Check sheet for the modelled part. Datum: model origin and axes. Units: mm. A direction names the side the tool comes from. Coordinates: 2 decimals unless noted, no trailing zeros. Order: outer loops, then holes, each group sorted by start corner. A loop starts at its lowest first (then second) coordinate and runs counter-clockwise, first axis right, second up. Notation, with made-up numbers: (-23.75, -27) -> (8.25, -27) arc R11 cw to (8.25, -8) -> close; hole circle Ø5 at (-25, 58). An arc over 180 degrees is marked (long way). Put each result on its own line as item: value. Start each with the question number.
```python
from build123d import *

# Parameters (mm, degrees)
SKETCH1_W           = 2.8
SKETCH1_H           = 2.8
SKETCH1_W_2         = 2.7
SKETCH1_H_2         = 2.7
BOSS_EXTRUDE1_DEPTH = 3


with BuildPart() as part:
    # Sketch1 → Boss-Extrude1 (new body)
    with BuildSketch(Plane(origin=(0, 0, 0), x_dir=(1, 0, 0), z_dir=(0, 1, 0))):
        with BuildLine():
            Line((-37.844649751, 18.090932989), (-37.844649751, 15.090932989))
            Line((-37.844649751, 15.090932989), (-35.044649751, 15.090932989))
            Line((-35.044649751, 15.090932989), (-35.044649751, 12.290932989))
            Line((-35.044649751, 12.290932989), (-37.844649751, 12.290932989))
            Line((-37.844649751, 12.290932989), (-37.844649751, 6.290932989))
            Line((-37.844649751, 6.290932989), (-35.344649751, 6.290932989))
            Line((-35.344649751, 6.290932989), (-35.344649751, -53.709067011))
            Line((-35.344649751, -53.709067011), (-37.844649751, -53.709067011))
            Line((-37.844649751, -53.709067011), (-37.844649751, -71.409067011))
            ThreePointArc((-37.844649751, -71.409067011), (-25.332467624, -76.857542339), (-11.813147026, -78.719948188))
            Line((-11.813147026, -78.719948188), (-8.844649751, -78.719948188))
            Line((-8.844649751, -78.719948188), (1.155350249, -78.719948188))
            Line((1.155350249, -78.719948188), (11.155350249, -78.719948188))
            Line((11.155350249, -78.719948188), (14.123847524, -78.719948188))
            ThreePointArc((14.123847524, -78.719948188), (27.643168122, -76.857542339), (40.155350249, -71.409067011))
            Line((40.155350249, -71.409067011), (40.155350249, -53.709067011))
            Line((40.155350249, -53.709067011), (37.655350249, -53.709067011))
            Line((37.655350249, -53.709067011), (37.655350249, 6.290932989))
            Line((37.655350249, 6.290932989), (40.155350249, 6.290932989))
            Line((40.155350249, 6.290932989), (40.155350249, 12.290932989))
            Line((40.155350249, 12.290932989), (37.355350249, 12.290932989))
            Line((37.355350249, 12.290932989), (37.355350249, 15.090932989))
            Line((37.355350249, 15.090932989), (40.155350249, 15.090932989))
            Line((40.155350249, 15.090932989), (40.155350249, 18.090932989))
            Line((40.155350249, 18.090932989), (-37.844649751, 18.090932989))
        make_face()
        Polygon((-35.567709863, -70.827218463), (-34.74906909, -68.149565146), (-32.071415773, -68.96820592), (-32.890056546, -71.645859236), align=None, mode=Mode.SUBTRACT)
        Polygon((-29.829881327, -72.581448691), (-29.011240554, -69.903795375), (-26.333587237, -70.722436148), (-27.15222801, -73.400089465), align=None, mode=Mode.SUBTRACT)
        Polygon((-14.857930166, -74.230896605), (-15.676570939, -76.908549921), (-18.354224255, -76.089909148), (-17.535583482, -73.412255831), align=None, mode=Mode.SUBTRACT)
        Polygon((-23.273412018, -71.658025603), (-20.595758701, -72.476666376), (-21.414399475, -75.154319693), (-24.092052791, -74.33567892), align=None, mode=Mode.SUBTRACT)
        Polygon((-33.489432073, -65.39759956), (-32.904688664, -63.484990048), (-13.778593544, -69.332424143), (-14.363336954, -71.245033655), align=None, mode=Mode.SUBTRACT)
        with Locations((-10.894649751, -75.619948559)):
            Rectangle(SKETCH1_W, SKETCH1_H, mode=Mode.SUBTRACT)
        with Locations((-4.894649751, -75.619948559)):
            Rectangle(SKETCH1_W, SKETCH1_H, mode=Mode.SUBTRACT)
        with Locations((-6.344649714, -67.869948559)):
            Rectangle(SKETCH1_W_2, SKETCH1_H_2, mode=Mode.SUBTRACT)
        Polygon((-29.732442135, -61.317767872), (-28.913801362, -58.640114555), (-26.236148045, -59.458755328), (-27.054788818, -62.136408645), align=None, mode=Mode.SUBTRACT)
        Polygon((-23.994613599, -63.0719981), (-23.175972826, -60.394344784), (-20.498319509, -61.212985557), (-21.316960283, -63.890638873), align=None, mode=Mode.SUBTRACT)
        Polygon((-17.055622388, -62.265523694), (-14.377969071, -63.084164467), (-15.196609844, -65.761817784), (-17.874263161, -64.94317701), align=None, mode=Mode.SUBTRACT)
        with Locations((1.205350249, -75.619949313)):
            Rectangle(SKETCH1_W, SKETCH1_H, mode=Mode.SUBTRACT)
        with Locations((-0.344649714, -67.869948559)):
            Rectangle(SKETCH1_W_2, SKETCH1_H_2, mode=Mode.SUBTRACT)
        with Locations((5.655350286, -67.869948559)):
            Rectangle(SKETCH1_W_2, SKETCH1_H_2, mode=Mode.SUBTRACT)
        with Locations((7.205350249, -75.619948559)):
            Rectangle(SKETCH1_W, SKETCH1_H, mode=Mode.SUBTRACT)
        with Locations((13.205350249, -75.619948559)):
            Rectangle(SKETCH1_W, SKETCH1_H, mode=Mode.SUBTRACT)
        Polygon((17.987271436, -76.908549921), (17.168630663, -74.230896605), (19.84628398, -73.412255831), (20.664924753, -76.089909148), align=None, mode=Mode.SUBTRACT)
        Polygon((23.725099972, -75.154319693), (22.906459199, -72.476666376), (25.584112516, -71.658025603), (26.402753289, -74.33567892), align=None, mode=Mode.SUBTRACT)
        Polygon((28.644287735, -70.722436148), (31.321941051, -69.903795375), (32.140581825, -72.581448691), (29.462928508, -73.400089465), align=None, mode=Mode.SUBTRACT)
        Polygon((34.38211627, -68.96820592), (37.059769587, -68.149565146), (37.87841036, -70.827218463), (35.200757044, -71.645859236), align=None, mode=Mode.SUBTRACT)
        with Locations((-30.644649751, 13.690932989)):
            Rectangle(SKETCH1_W, SKETCH1_H, mode=Mode.SUBTRACT)
        with Locations((32.955350249, 13.690932989)):
            Rectangle(SKETCH1_W, SKETCH1_H, mode=Mode.SUBTRACT)
    extrude(amount=BOSS_EXTRUDE1_DEPTH)


solid = part.part
```
1) Sectioned sample at A-A (y = 1.8). State how many separate pieces and enclosed holes the cut face has, plus the area to 3 significant figures.
2) Access from +Z, -Z, +X, -X, +Y, -Y to the whole of each face (thin tool, end or side, straight path). Record for faces 4 (the flat face through (-36, 1, -12.291)), 5 (the flat face through (4.305, 1, 68)), 6 (the flat face through (39, 1, 53.709)).
3) Sectioned sample at B-B (z = 48). Record the boundary of the cut face in (x, y), plus the area to 3 significant figures.
4) Scan lines: line 1 along Z through (x, y) = (6, 2.35); line 2 along Z through (x, y) = (5.5, 0.3); line 3 along Z through (x, y) = (7.5, 2.65). Record each from-to range of solid material in increasing order. Write a range as [from, to].
5) Mould release check, pull along X, two halves, no side actions. Record for faces 1 (the flat face through (1, 1, 78.72)), 2 (the flat face through (11.805, 1, 76)), 3 (the cylindrical face through (-25.517, 1.479, 76.805)): +X half, -X half, draft (parallel to the pull), parting line (faces both ways), or undercut.
6) Gauge pin test, flat ends, axial feed: pin 1 (1.4 mm diameter, centred on y = 2, z = 75.5, fed in from -X); pin 2 (0.9 mm diameter, centred on y = 2, z = 33, fed in from +X); pin 3 (1.4 mm diameter, centred on x = -36.5, y = 2, fed in from +Z). Record the tip position at first contact, or that the pin passes through.
Entries:
1. separate pieces: 1
1. enclosed holes: 22
1. area: 6,910 mm2
2. face 4: -X, +Y, -Y
2. face 5: +Y, -Y
2. face 6: +X, +Y, -Y
3. outline: (-35.34, 0) -> (37.66, 0) -> (37.66, 3) -> (-35.34, 3) -> close
3. area: 219 mm2
4. line 1: z = [-18.09, 66.52], [69.22, 74.22], [77.02, 78.72]
4. line 2: z = [-18.09, 66.52], [69.22, 78.72]
4. line 3: z = [-18.09, 74.22], [77.02, 78.72]
5. face 1: draft
5. face 2: undercut
5. face 3: -X half
6. pin 1: stops at x = -31.22
6. pin 2: stops at x = 37.66
6. pin 3: stops at z = 72.59
